Can you work these out from the model? Positions are in its coordinate system, mm. A direction names the side the tool comes from. Round coordinates to 2 decimals unless told otherwise and drop trailing zeros. Loops run counter-clockwise (first coordinate to the right, second up) from the corner with the lowest first, then second, coordinate; pieces in that order, holes last. Notation, with made-up numbers: M -27.75,6.5 L -19.75,6.5 A25 cw -19.75,18.5 Z; hole C -37,-17 d7. An arc over 180 degrees is marked long. Use a Markdown table: item, result. Add a question column.
```python
from build123d import *

# Parameters (mm, degrees)
F0_W     = 100
F0_H     = 11
F1_DEPTH = 20
F2_W     = 100
F2_H     = 5
F3_DEPTH = 8
F4_R     = 2.99999


# Not quite as in the source:
# - a fillet or chamfer is up to 0.001 mm smaller than in the source, because OpenCascade refuses the exact size


with BuildPart() as f1:
    # F0 (on Front) → F1 (new body)
    with BuildSketch(Plane.XZ):
        Rectangle(F0_W, F0_H)
    extrude(amount=-F1_DEPTH)

    # F2 (on face) → F3 (cut)
    with BuildSketch(Plane.XZ):
        Rectangle(F2_W, F2_H)
    extrude(amount=-F3_DEPTH, mode=Mode.SUBTRACT)

    # F4 (radius 3 in the source; OpenCascade refuses exactly that, so slightly less here)
    f4_edges = [f1.edges().sort_by_distance(p)[0] for p in [
        (0, 20, 5.5),
        (0, 20, -5.5),
        (0, 0, 5.5),
        (0, 0, -5.5),
    ]]
    fillet(f4_edges, radius=F4_R)


solid = f1.part
```
(1) I'm going to push flat-ended pins straight in: pin 1 (9 mm diameter, centred on x = 23.5, y = 2.5, fed in from +Z); pin 2 (1 mm diameter, centred on x = 17, z = 1.5, fed in from -Y). Where does each tip first touch, or does it pass through?
(2) Suppose I cut it at C-C on z = -1.25. List the corners of the cut face in (x, y) for me.
(3) On a 3-axis mill with a long thin cutter (end or side, diameter ignored), from which of +Z, -Z, +X, -X, +Y, -Y can I reach the whole of each face in a straight line? I mean faces 5 (the face through (-1, 10, -5.5)), 6 (the face through (-1, 4, -2.5)). Say none if no direction works.
(4) Thinking about a two-plate mould opening in Z: for faces 1 (the face through (0.7, 0.86, -4.6)), 2 (the face through (50, 12, 0)), 3 (the face through (-1, 4, 2.5)), 4 (the face through (0.7, 19.1, 4.64)), which applies, released by +Z, released by -Z, zero draft, split by the parting line, or undercut?
(5) Suppose I cut it at D-D on z = 4.5. List the corners of the cut face in (x, y) for me, and give its area (3 significant figures).
(6) Suppose I cut it at A-A on y = 5.75. List the corners of the cut face in (x, z) for me, and give its area (3 significant figures).
(7) If I drill on probe 1 along Z at (x, y) = (-28, 6.5); probe 2 along Y at (x, z) = (41.5, -0.25); probe 3 along Y at (x, z) = (19.5, -4.75), over which ranges is the centre line in solid material (lowest first)? Write a range as [from, to].
Results below:
| question | item | result |
|---|---|---|
| 1 | pin 1 | stops at z = 5.5 |
| 1 | pin 2 | stops at y = 8 |
| 2 | outline | M -50,8 L 50,8 L 50,20 L -50,20 Z |
| 3 | face 5 | -Z, +X, -X, +Y, -Y |
| 3 | face 6 | +X, -X, -Y |
| 4 | face 1 | released by -Z |
| 4 | face 2 | zero draft |
| 4 | face 3 | undercut |
| 4 | face 4 | released by +Z |
| 5 | outline | M -50,0.76 L 50,0.76 L 50,19.24 L -50,19.24 Z |
| 5 | area | 1,850 mm² |
| 6 | outline | M -50,-5.5 L 50,-5.5 L 50,-2.5 L -50,-2.5 Z; M -50,2.5 L 50,2.5 L 50,5.5 L -50,5.5 Z |
| 6 | area | 600 mm² |
| 7 | probe 1 | z = [-5.5, -2.5], [2.5, 5.5] |
| 7 | probe 2 | y = [8, 20] |
| 7 | probe 3 | y = [1.02, 18.98] |
